Design review of the part shown in the three views and the two pictorial views. Dimensions are in mm from the part's minimum x, y and z. Coordinates: 2 decimals unless noted, no trailing zeros. Write each loop counter-clockwise with the first axis right and the second up, starting at its lowest first coordinate (ties: lowest second). Pieces come first, ordered by that corner, then holes. Notation, with made-up numbers: (27.5, 46) - (52.5, 46) arc R11 ccw to (52.5, 55) - close; hole circle Ø10 at (33, 44). An arc over 180 degrees is marked (long way). Return JSON: item names as keys, results as strings. Group by question number.
(1) We need section C-C on z = 40.5. State the section outline as (x, y) points (3 decimals), then the cut area to 3 significant figures.
(2) To check wall thickness, follow L1, parallel to Y at x = 1.2, z = 40.5; L2, parallel to Y at x = 2.2, z = 59; L3, parallel to Y at x = 0.2, z = 51. State the ranges of each line that lie inside material, in increasing order. Write a range as from..to.
(3) We need section B-B on x = 0.7. State the section outline as (y, z) points (3 decimals).
(4) We need section A-A on y = 127. State the section outline as (x, z) points (3 decimals), then the cut area to 3 significant figures.
(5) For pin 1 Ø14.5 at (y, z) = (127, 41.275) entering from -X, flat-tipped, find the tip position at first contact; note if it passes through.
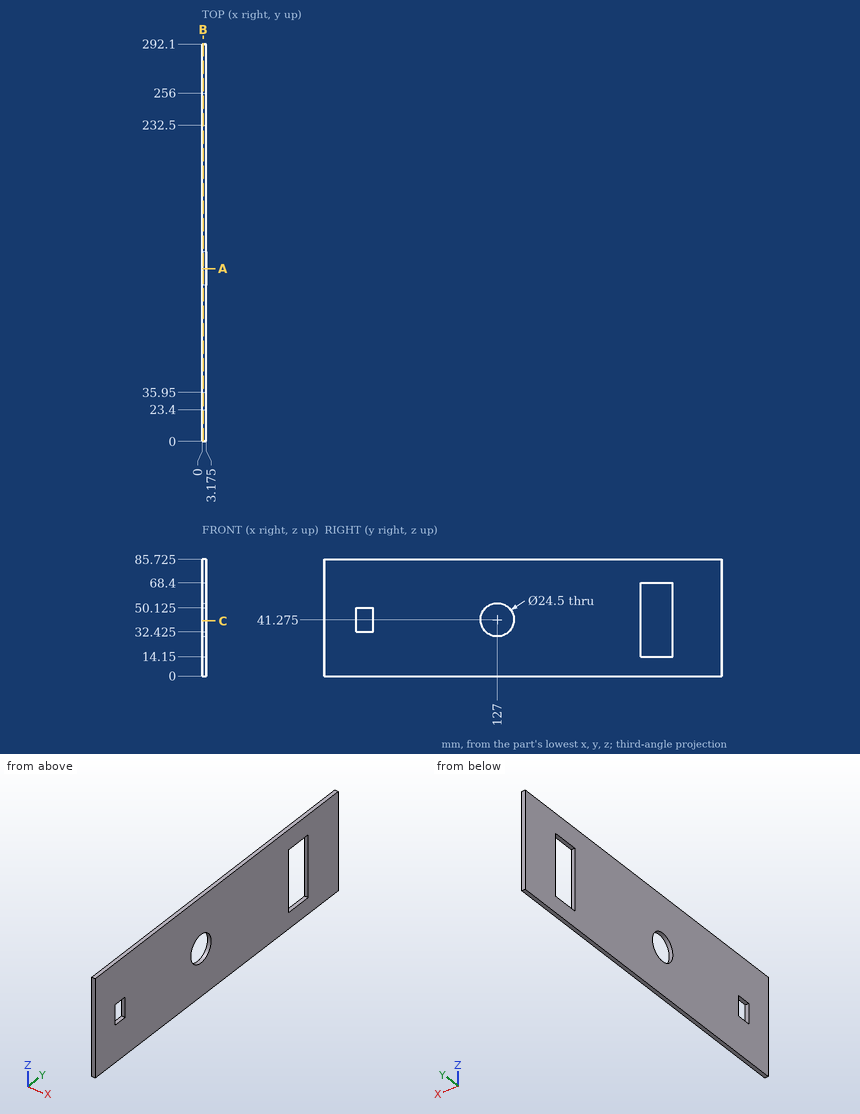
Ans:
{
 "1": {"outline": "(0, 0) - (3.175, 0) - (3.175, 23.4) - (0, 23.4) - close; (0, 35.95) - (3.175, 35.95) - (3.175, 114.775) - (0, 114.775) - close; (0, 139.225) - (3.175, 139.225) - (3.175, 232.5) - (0, 232.5) - close; (0, 256) - (3.175, 256) - (3.175, 292.1) - (0, 292.1) - close", "area": "735 mm²"},
 "2": {"L1": "0..23.4, 35.95..114.77, 139.23..232.5, 256..292.1", "L2": "0..232.5, 256..292.1", "L3": "0..119.55, 134.45..232.5, 256..292.1"},
 "3": {"outline": "(0, 0) - (292.1, 0) - (292.1, 85.725) - (0, 85.725) - close; hole (23.4, 32.425) - (35.95, 32.425) - (35.95, 50.125) - (23.4, 50.125) - close; hole circle Ø24.5 at (127, 41.275); hole (232.5, 14.15) - (256, 14.15) - (256, 68.4) - (232.5, 68.4) - close"},
 "4": {"outline": "(0, 0) - (3.175, 0) - (3.175, 29.025) - (0, 29.025) - close; (0, 53.525) - (3.175, 53.525) - (3.175, 85.725) - (0, 85.725) - close", "area": "194 mm²"},
 "5": {"pin 1": "through"}
}
